Here's how the part is built. I have some questions about the finished solid (model axes, mm). Face numbers are marked on the shaded views. Round coordinates to 2 decimals unless told otherwise and drop trailing zeros. Order: outer loops, then holes, each group sorted by start corner. A loop starts at its lowest first (then second) coordinate and runs counter-clockwise, first axis right, second up. Notation, with made-up numbers: (-15, -23.75) - (35, -23.75) arc R13 cw to (35, -17.75) - close; hole circle Ø6 at (74.25, 56.25). An arc over 180 degrees is marked (long way). One line per item, written item: value.
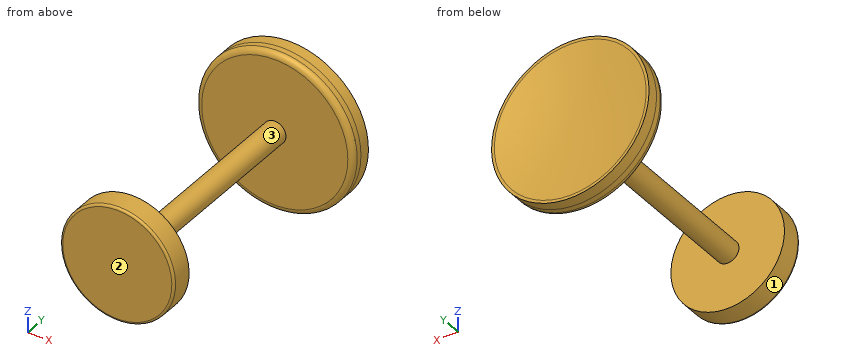
from build123d import *

# Parameters (mm, degrees)
SKETCH1_R           = 17.78
BOSS_EXTRUDE1_DEPTH = 2.54
FILLET1_R           = 0.508
FILLET2_R           = 1.27


with BuildPart() as part:
    # Sketch1 → Boss-Extrude1 (new body)
    with BuildSketch(Plane(origin=(0, 0, 0), x_dir=(1, 0, 0), z_dir=(0, 1, 0))):
        Circle(SKETCH1_R)
    extrude(amount=BOSS_EXTRUDE1_DEPTH)

    # Sketch2 → Revolve1 (revolve)
    with BuildSketch(Plane(origin=(0, 0, 0), x_dir=(0, 0, -1), z_dir=(1, 0, 0))):
        with BuildLine():
            Line((-17.78, 2.54), (-17.78, 5.08))
            Line((-17.78, 5.08), (-17.145, 5.08))
            ThreePointArc((-17.145, 5.08), (-8.625254344, 3.652710903), (0, 3.175))
            Line((0, 3.175), (0, 2.54))
            Line((0, 2.54), (-17.78, 2.54))
        make_face()
        Polygon((0, 0), (0, -53.34), (-12.827, -53.34), (-12.827, -48.26), (-2.54, -48.26), (-2.54, 0), align=None)
    revolve(axis=Axis((0, 0, 0), (0, -1, 0)))

    # Fillet1
    fillet1_edges = [part.edges().sort_by_distance(p)[0] for p in [
        (0, -53.34, -12.827),
    ]]
    fillet(fillet1_edges, radius=FILLET1_R)

    # Fillet2
    fillet2_edges = [part.edges().sort_by_distance(p)[0] for p in [
        (-17.78, 0, 0),
    ]]
    fillet(fillet2_edges, radius=FILLET2_R)


solid = part.part
Q1. If I drill on line 1 along Z through (x, y) = (0, -22.5); line 2 along Y through (x, z) = (11.5, 4); line 3 along Y through (x, z) = (9.5, 6.5), over which ranges is the centre line in solid material (lowest first)?
Results list:
line 1: -2.54 to 2.54
line 2: -53.34 to -48.26, 0 to 4.13
line 3: -53.34 to -48.26, 0 to 4.03
Q2. We'd pull the mould along Y, two halves only. Please class the marked faces 1, 2 and 3: released by +Y, released by -Y, zero draft, split by the parting line, or undercut.
Results list:
face 1: zero draft
face 2: released by -Y
face 3: undercut
Q3. If we section it at B-B, the plane x = 0: Please give me the cut outline in (y, z) (3 decimals), then the cut area to 3 significant figures.
Results list:
outline: (-53.34, -12.319) arc R0.508 ccw to (-52.832, -12.827) - (-48.26, -12.827) - (-48.26, -2.54) - (0, -2.54) - (0, -16.51) arc R1.27 ccw to (1.27, -17.78) - (5.08, -17.78) - (5.08, -17.145) arc R78.105 cw to (5.08, 17.145) - (5.08, 17.78) - (1.27, 17.78) arc R1.27 ccw to (0, 16.51) - (0, 2.54) - (-48.26, 2.54) - (-48.26, 12.827) - (-52.832, 12.827) arc R0.508 ccw to (-53.34, 12.319) - close
area: 512 mm²
Q4. Will these pins go through, and if not, where does the flat tip stop? pin 1 (3 mm diameter, centred on y = -37.5, z = -3.5, fed in from +X); pin 2 (5 mm diameter, centred on y = -9.5, z = 2, fed in from -X); pin 3 (5 mm diameter, centred on x = -0.5, y = -23.5, fed in from +Z).
Results list:
pin 1: x = 1.57
pin 2: x = -2.54
pin 3: z = 2.54
Q5. If we section it at C-C, the plane y = -13: Please give me the cut outline in (x, z), then the cut area to 3 significant figures.
Results list:
outline: circle Ø5.08 at (0, 0)
area: 20.3 mm²
Q6. If we section it at A-A, the plane z = 0: Please give me the cut outline in (x, y) (3 decimals).
Results list:
outline: (-17.78, 1.27) arc R1.27 ccw to (-16.51, 0) - (-2.54, 0) - (-2.54, -48.26) - (-12.827, -48.26) - (-12.827, -52.832) arc R0.508 ccw to (-12.319, -53.34) - (12.319, -53.34) arc R0.508 ccw to (12.827, -52.832) - (12.827, -48.26) - (2.54, -48.26) - (2.54, 0) - (16.51, 0) arc R1.27 ccw to (17.78, 1.27) - (17.78, 5.08) - (17.145, 5.08) arc R78.105 cw to (-17.145, 5.08) - (-17.78, 5.08) - close
